Check sheet for the modelled part. Datum: model origin and axes. Units: mm. Face numbers are marked on the shaded views. A direction names the side the tool comes from. Round coordinates to 2 decimals unless told otherwise and drop trailing zeros. Order: outer loops, then holes, each group sorted by start corner. A loop starts at its lowest first (then second) coordinate and runs counter-clockwise, first axis right, second up.
(1) Sectioned sample at C-C, the plane z = -86.5. Enter the section's corners in (x, y), and give its area (3 significant figures).
(2) Sectioned sample at B-B, the plane x = 29. Enter the section's corners in (y, z).
(3) Sectioned sample at A-A, the plane y = 1.75. Enter the section's corners in (x, z) (3 decimals).
(4) Thickness scan on probe 1 along Z at (x, y) = (4, 16.5); probe 2 along X at (y, z) = (14.5, -106); probe 3 along Z at (x, y) = (-11, 10.75). Record the ranges inside material, lowest first.
(5) Depth check by flat-ended pin: pin 1 (6 mm diameter, centred on x = -22, y = 6, fed in from -Z); pin 2 (5 mm diameter, centred on x = 47.5, y = 5.5, fed in from -Z); pin 3 (4 mm diameter, centred on y = 15, z = -52, fed in from +X). Enter the tip coordinate at first touch or a pass-through.
(6) Tool access check on the marked faces 1 and 2. Record the directions out of +Z, -Z, +X, -X, +Y, -Y that give a thin tool (end or side, any length) a straight path to the whole face; none if there is none.
Autodesk Inventor part; units mm, degrees
ref_plane "YZ Plane" through (0, 0, 0) normal (1, 0, 0) x (0, 1, 0)
ref_plane "XZ Plane" through (0, 0, 0) normal (0, 1, 0) x (-1, 0, 0)
ref_plane "XY Plane" through (0, 0, 0) normal (0, 0, 1) x (1, 0, 0)
sketch "Sketch1" plane through (0, 0, 0) normal (0, 1, 0) x (-1, 0, 0)
  line L0 (0, 0) -> (67.8242, -117.475)
  line L1 (0, 0) -> (135.6484, 0) construction
  line L2 (67.8242, -117.475) -> (62.325, -120.65)
  line L3 (62.325, -120.65) -> (-3.6662, -6.35)
  line L4 (-0.56, 0) -> (-73.5162, 0)
  line L5 (-73.5162, 0) -> (-73.5162, -6.35)
  line L6 (-3.6662, -6.35) -> (-73.5162, -6.35)
  line L7 (0, 0) -> (-0.56, 0)
  dimension "d0" = 60
  dimension "d2" = 6.35
  dimension "d3" = 6.35
  dimension "d4" = 0
  dimension "d5" = 114.3
  dimension "d6" = 69.85
extrude "Extrusion1" add sketch "Sketch1" along normal blind 19.05
sketch "Sketch2" plane through (0, 0, 0) normal (0, 0, 1) x (1, 0, 0)
  line L0 (73.5162, 0) -> (0, 0)
  line L1 (73.5162, 0) -> (73.5162, 19.05)
  line L2 (0, 19.05) -> (73.5162, 19.05)
  line L3 (0, 0) -> (0, 19.05)
  point P0 (67.1662, 9.525)
  point P1 (54.4662, 9.525)
  dimension "d9" = 6.35
  dimension "d10" = 19.05
  dimension "d11" = 9.525
  dimension "d12" = 9.525
hole "Hole1" at (67.1662, 9.525, 0) at (54.4662, 9.525, 0) direction (0, 0, -1) diameter 4.445 end through all
sketch "Sketch3" plane through (0, 0, 0) normal (-0.8660254, 0, 0.5) x (0.5, 0, 0.8660254)
  line L0 (0, 0) -> (-135.6484, 0)
  line L1 (0, 0) -> (0, 19.05)
  line L2 (-135.6484, 19.05) -> (0, 19.05)
  line L3 (-135.6484, 0) -> (-135.6484, 19.05)
  point P0 (-129.2984, 9.525)
  point P1 (-91.1984, 9.525)
  dimension "d20" = 6.35
  dimension "d21" = 44.45
  dimension "d22" = 9.525
  dimension "d23" = 9.525
hole "Hole2" at (-64.6492, 9.525, -111.9757) at (-45.5992, 9.525, -78.9802) direction (0.8660254, 0, -0.5) diameter 4.064 end through all
properties part number "CollectionAngleBracket"
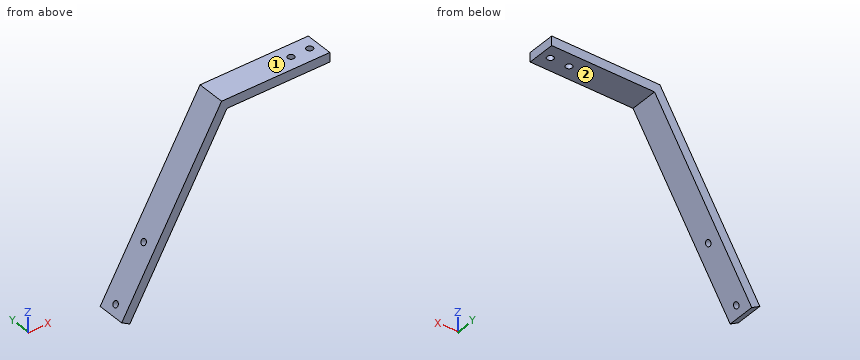
Derived:
1. outline: (-49.94, 0) - (-42.61, 0) - (-42.61, 19.05) - (-49.94, 19.05) - close
1. area: 140 mm2
2. outline: (0, -6.35) - (19.05, -6.35) - (19.05, 0) - (0, 0) - close
3. outline: (-67.824, -117.475) - (-62.325, -120.65) - (3.666, -6.35) - (73.516, -6.35) - (73.516, 0) - (0, 0) - close
4. probe 1: z = -6.35 to 0
4. probe 2: x = -61.2 to -53.87
4. probe 3: z = -31.75 to -19.05
5. pin 1: stops at z = -56
5. pin 2: stops at z = -6.35
5. pin 3: stops at x = -21.54
6. face 1: +Z, +X, -X, +Y, -Y
6. face 2: -Z, +X, +Y, -Y
